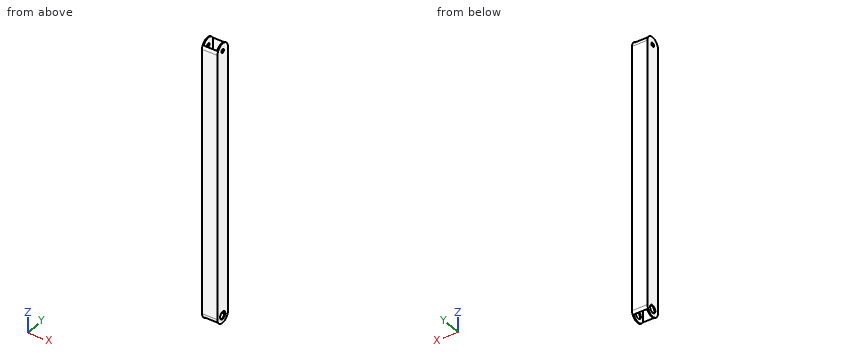
```python
from build123d import *

# Parameters (mm, degrees)
SKETCH1_W           = 25.4
SKETCH1_H           = 25.4
SKETCH1_W_2         = 22.225
SKETCH1_H_2         = 22.225
BOSS_EXTRUDE1_DEPTH = 473.2274
CUT_EXTRUDE1_DEPTH  = 26.4
SKETCH3_R           = 3.175
SKETCH3_R_2         = 6.35
CUT_EXTRUDE2_DEPTH  = 26.4
CUT_EXTRUDE3_DEPTH  = 26.4


with BuildPart() as part:
    # Sketch1 → Boss-Extrude1 (new body)
    with BuildSketch(Plane.XY):
        Rectangle(SKETCH1_W, SKETCH1_H)
        Rectangle(SKETCH1_W_2, SKETCH1_H_2, mode=Mode.SUBTRACT)
    extrude(amount=BOSS_EXTRUDE1_DEPTH)

    # Sketch2 → Cut-Extrude1 (cut, through all)
    with BuildSketch(Plane(origin=(12.7, 0, 0), x_dir=(0, 0, -1), z_dir=(1, 0, 0))):
        with BuildLine():
            Line((-460.5274, 12.7), (-473.2274, 12.7))
            Line((-473.2274, 12.7), (-473.2274, 9.7e-08))
            ThreePointArc((-473.2274, 9.7e-08), (-469.507656087, 8.980256155), (-460.5274, 12.7))
        make_face()
        with BuildLine():
            ThreePointArc((-460.5274, -12.7), (-469.507656155, -8.980256087), (-473.2274, 9.7e-08))
            Line((-473.2274, 9.7e-08), (-473.2274, -12.7))
            Line((-473.2274, -12.7), (-460.5274, -12.7))
        make_face()
    extrude(amount=-CUT_EXTRUDE1_DEPTH, mode=Mode.SUBTRACT)

    # Sketch3 → Cut-Extrude2 (cut, through all)
    with BuildSketch(Plane(origin=(12.7, 0, 0), x_dir=(0, 0, -1), z_dir=(1, 0, 0))):
        with Locations((-460.5274, 0)):
            Circle(SKETCH3_R)
        with Locations((-12.7, 0)):
            Circle(SKETCH3_R_2)
    extrude(amount=-CUT_EXTRUDE2_DEPTH, mode=Mode.SUBTRACT)

    # Sketch5 → Cut-Extrude3 (cut, through all)
    with BuildSketch(Plane(origin=(12.7, 0, 0), x_dir=(0, 0, -1), z_dir=(1, 0, 0))):
        with BuildLine():
            Line((0, 12.7), (-12.7, 12.7))
            ThreePointArc((-12.7, 12.7), (-3.719743879, 8.980256121), (0, 0))
            Line((0, 0), (0, 12.7))
        make_face()
        with BuildLine():
            Line((0, -12.7), (0, 0))
            ThreePointArc((0, 0), (-3.719743879, -8.980256121), (-12.7, -12.7))
            Line((-12.7, -12.7), (0, -12.7))
        make_face()
    extrude(amount=-CUT_EXTRUDE3_DEPTH, mode=Mode.SUBTRACT)


solid = part.part
```
Here's how the part is built. I have some questions about the finished solid (model axes, mm). Give positions to 0.01 mm unless a question says otherwise; leave off trailing zeros. Loops run counter-clockwise (first coordinate to the right, second up) from the corner with the lowest first, then second, coordinate; pieces in that order, holes last. Notation, with made-up numbers: M 1.5,-9.75 L 54.5,-9.75 A16 cw 54.5,11.25 Z; hole C 82.5,23 d5. An arc over 180 degrees is marked long. Use one line per item in the form item = value. Start each with the question number.
Q1. If we section it at B-B (x = 4): Write out the boundary of the cut face in (y, z).
Q2. I need wall thicknesses on line 1 along Y through (x, z) = (3.25, 74); line 2 along Y through (x, z) = (-11.45, 12.7). Which ranges of each line are inside material? Lowest first, please.
Q3. Will this pin go through, and if not, where does the flat tip stop? pin 1 Ø11.5 at (y, z) = (0, 12.7) entering from -X.
Q4. If we section it at A-A (z = 148): Write out the boundary of the cut face in (x, y).
Taken from the geometry:
q1.outline = M -12.7,12.7 A12.7 ccw -11.11,6.55 L -11.11,466.68 A12.7 ccw -12.7,460.53 Z; M 11.11,6.55 A12.7 ccw 12.7,12.7 L 12.7,460.53 A12.7 ccw 11.11,466.68 Z
q2.line_1 = -12.7 to -11.11, 11.11 to 12.7
q2.line_2 = -12.7 to -6.35, 6.35 to 12.7
q3.pin_1 = through
q4.outline = M -12.7,-12.7 L 12.7,-12.7 L 12.7,12.7 L -12.7,12.7 Z; hole M -11.11,-11.11 L 11.11,-11.11 L 11.11,11.11 L -11.11,11.11 Z
